Here's how the part is built. I have some questions about the finished solid (model axes, mm). A direction names the side the tool comes from. Round coordinates to 2 decimals unless told otherwise and drop trailing zeros. Order: outer loops, then holes, each group sorted by start corner. A loop starts at its lowest first (then second) coordinate and runs counter-clockwise, first axis right, second up.
Solid Edge part; units mm, degrees
sketch "Sketch1" plane through (0, 0, 0) normal (0, 0, 1) x (1, 0, 0)
  arc A0 (-0.5843, 4.4447) -> (0, 5.0777) centre (0.0507, 4.4447) cw
  arc A1 (0.5843, 4.4447) -> (0, 5.0777) centre (-0.0507, 4.4447) ccw
  line L0 (0.5843, 3.7649) -> (0.5843, 4.4447)
  arc A2 (2.249, 3.0754) -> (0.5843, 3.7649) centre (0, 0) ccw
  line L1 (2.249, 3.0754) -> (2.7297, 3.5561)
  arc A3 (2.7297, 3.5561) -> (3.5905, 3.5905) centre (3.1787, 3.1071) cw
  arc A4 (3.5561, 2.7297) -> (3.5905, 3.5905) centre (3.1071, 3.1787) ccw
  line L2 (3.0754, 2.249) -> (3.5561, 2.7297)
  arc A5 (3.7649, 0.5843) -> (3.0754, 2.249) centre (0, 0) ccw
  line L3 (3.7649, 0.5843) -> (4.4447, 0.5843)
  arc A6 (4.4447, 0.5843) -> (5.0777, 0) centre (4.4447, -0.0507) cw
  arc A7 (4.4447, -0.5843) -> (5.0777, 0) centre (4.4447, 0.0507) ccw
  line L4 (3.7689, -0.5843) -> (4.4447, -0.5843)
  line L5 (3.7625, -0.5998) -> (3.7689, -0.5843)
  arc A8 (3.7625, -0.5998) -> (3.0754, -2.249) centre (0, 0) cw
  line L6 (3.0754, -2.249) -> (3.5561, -2.7297)
  arc A9 (3.5561, -2.7297) -> (3.5905, -3.5905) centre (3.1071, -3.1787) cw
  arc A10 (2.7297, -3.5561) -> (3.5905, -3.5905) centre (3.1787, -3.1071) ccw
  line L7 (2.249, -3.0754) -> (2.7297, -3.5561)
  arc A11 (2.249, -3.0754) -> (0.5843, -3.7649) centre (0, 0) cw
  line L8 (0.5843, -3.7649) -> (0.5843, -4.4447)
  arc A12 (0.5843, -4.4447) -> (0, -5.0777) centre (-0.0507, -4.4447) cw
  arc A13 (-0.5843, -4.4447) -> (0, -5.0777) centre (0.0507, -4.4447) ccw
  line L9 (-0.5843, -3.7649) -> (-0.5843, -4.4447)
  arc A14 (-0.5843, -3.7649) -> (-2.249, -3.0754) centre (0, 0) cw
  line L10 (-2.249, -3.0754) -> (-2.7297, -3.5561)
  arc A15 (-2.7297, -3.5561) -> (-3.5905, -3.5905) centre (-3.1787, -3.1071) cw
  arc A16 (-3.5561, -2.7297) -> (-3.5905, -3.5905) centre (-3.1071, -3.1787) ccw
  line L11 (-3.0754, -2.249) -> (-3.5561, -2.7297)
  arc A17 (-3.0754, -2.249) -> (-3.7649, -0.5843) centre (0, 0) cw
  line L12 (-3.7649, -0.5843) -> (-4.4447, -0.5843)
  arc A18 (-4.4447, -0.5843) -> (-5.0777, 0) centre (-4.4447, 0.0507) cw
  arc A19 (-4.4447, 0.5843) -> (-5.0777, 0) centre (-4.4447, -0.0507) ccw
  line L13 (-3.7649, 0.5843) -> (-4.4447, 0.5843)
  arc A20 (-3.7649, 0.5843) -> (-3.0754, 2.249) centre (0, 0) cw
  line L14 (-3.0754, 2.249) -> (-3.5561, 2.7297)
  arc A21 (-3.5561, 2.7297) -> (-3.5905, 3.5905) centre (-3.1071, 3.1787) cw
  arc A22 (-2.7297, 3.5561) -> (-3.5905, 3.5905) centre (-3.1787, 3.1071) ccw
  line L15 (-2.249, 3.0754) -> (-2.7297, 3.5561)
  arc A23 (-2.249, 3.0754) -> (-0.5843, 3.7649) centre (0, 0) cw
  line L16 (-0.5843, 3.7649) -> (-0.5843, 4.4447)
extrude "Protrusion1" add sketch "Sketch1" along normal mid plane 6.35
sketch "Sketch2" plane through (0, 0, 0) normal (0, 0, 1) x (1, 0, 0)
  arc A0 (3.5561, 2.7297) -> (3.5905, 3.5905) centre (3.1071, 3.1787) ccw
  arc A1 (2.7297, 3.5561) -> (3.5905, 3.5905) centre (3.1787, 3.1071) cw
  arc A2 (3.5561, 2.7297) -> (2.7297, 3.5561) centre (3.1429, 3.1429) cw
  arc A3 (4.4447, 0.5843) -> (4.4447, -0.5843) centre (4.4447, 0) ccw
  arc A4 (4.4447, -0.5843) -> (5.0777, 0) centre (4.4447, 0.0507) ccw
  arc A5 (4.4447, 0.5843) -> (5.0777, 0) centre (4.4447, -0.0507) cw
  arc A6 (3.5561, -2.7297) -> (2.7297, -3.5561) centre (3.1429, -3.1429) ccw
  arc A7 (2.7297, -3.5561) -> (3.5905, -3.5905) centre (3.1787, -3.1071) ccw
  arc A8 (3.5561, -2.7297) -> (3.5905, -3.5905) centre (3.1071, -3.1787) cw
  arc A9 (0.5843, -4.4447) -> (0, -5.0777) centre (-0.0507, -4.4447) cw
  arc A10 (-0.5843, -4.4447) -> (0, -5.0777) centre (0.0507, -4.4447) ccw
  arc A11 (0.5843, -4.4447) -> (-0.5843, -4.4447) centre (0, -4.4447) ccw
  arc A12 (-2.7297, -3.5561) -> (-3.5561, -2.7297) centre (-3.1429, -3.1429) ccw
  arc A13 (-3.5561, -2.7297) -> (-3.5905, -3.5905) centre (-3.1071, -3.1787) ccw
  arc A14 (-2.7297, -3.5561) -> (-3.5905, -3.5905) centre (-3.1787, -3.1071) cw
  arc A15 (-4.4447, 0.5843) -> (-4.4447, -0.5843) centre (-4.4447, 0) cw
  arc A16 (-4.4447, -0.5843) -> (-5.0777, 0) centre (-4.4447, 0.0507) cw
  arc A17 (-4.4447, 0.5843) -> (-5.0777, 0) centre (-4.4447, -0.0507) ccw
  arc A18 (-2.7297, 3.5561) -> (-3.5905, 3.5905) centre (-3.1787, 3.1071) ccw
  arc A19 (-3.5561, 2.7297) -> (-3.5905, 3.5905) centre (-3.1071, 3.1787) cw
  arc A20 (-2.7297, 3.5561) -> (-3.5561, 2.7297) centre (-3.1429, 3.1429) cw
  arc A21 (0.5843, 4.4447) -> (-0.5843, 4.4447) centre (0, 4.4447) cw
  arc A22 (-0.5843, 4.4447) -> (0, 5.0777) centre (0.0507, 4.4447) cw
  arc A23 (0.5843, 4.4447) -> (0, 5.0777) centre (-0.0507, 4.4447) ccw
extrude "ExtrudedProtrusion_2" add sketch "Sketch2" against normal blind 4.445
sketch "Sketch3" plane through (0, 0, -3.175) normal (0, 0, -1) x (0, 1, 0)
  circle A0 centre (0, 0) radius 0.2794
extrude "Cutout1" cut sketch "Sketch3" against normal blind 26.4035
1. I'm going to push flat-ended pins straight in: P1, Ø1.5, axis at y = 4, z = -1.5, coming from the -X side; P2, Ø1.5, axis at x = 1, z = -0.5, coming from the -Y side; P3, Ø0.5, axis at y = -4.5, z = 0, coming from the +X side. Where does each tip first touch, or does it pass through?
Evaluation:
P1: stops at x = -3.74
P2: stops at y = -5
P3: stops at x = 0.58
2. If we section it at C-C, the plane y = -2: Write out the boundary of the cut face in (x, z) (3 decimals), and give its area (3 significant figures).
Evaluation:
outline: (-3.243, -3.175) - (3.243, -3.175) - (3.243, 3.175) - (-3.243, 3.175) - close
area: 41.2 mm2
3. If we section it at A-A, the plane y = 3.25: Write out the boundary of the cut face in (x, z) (3 decimals).
Evaluation:
outline: (-3.738, -4.445) - (-2.568, -4.445) - (-2.568, -3.175) - (-2.424, -3.175) - (-2.424, 3.175) - (-3.738, 3.175) - close; (-1.988, -3.175) - (1.988, -3.175) - (1.988, 3.175) - (-1.988, 3.175) - close; (2.424, -3.175) - (2.568, -3.175) - (2.568, -4.445) - (3.738, -4.445) - (3.738, 3.175) - (2.424, 3.175) - close
4. I need wall thicknesses on probe 1 along X at (y, z) = (0, -1.5); probe 2 along Z at (x, y) = (2.5, 2.5) (3 decimals); probe 3 along X at (y, z) = (4.5, -1.5). Which ranges of each line are inside material? Lowest first, please.
Evaluation:
probe 1: x = -5.08 to -0.28, 0.28 to 5.08
probe 2: z = -3.175 to 3.175
probe 3: x = -0.58 to 0.58
5. If we mould it in two halves opening along Y, with no side actions, what happens to faces 4 (the cylindrical face through (-3.74, 3.15, -0.69)), 5 (the cylindrical face through (3.86, 0.01, -3.8)), 6 (the flat face through (-3, -3, -4.445))? For each: released by +Y, released by -Y, zero draft, split by the parting line, or undercut.
Evaluation:
face 4: undercut
face 5: split by the parting line
face 6: zero draft
6. On a 3-axis mill with a long thin cutter (end or side, diameter ignored), from which of +Z, -Z, +X, -X, +Y, -Y can I reach the whole of each face in a straight line? I mean faces 1 (the cylindrical face through (-2.74, 2.72, -3.8)), 2 (the cylindrical face through (-1.47, 3.515, -0.044)), 3 (the cylindrical face through (-1.446, -3.525, -0.044)). Say none if no direction works.
Evaluation:
face 1: -Z
face 2: +Z, -Z, +Y
face 3: +Z, -Z, -Y
7. If we section it at B-B, the plane x = 4: Write out the boundary of the cut face in (y, z) (3 decimals), and give its area (3 significant figures).
Evaluation:
outline: (-0.584, -3.175) - (-0.379, -3.175) - (-0.379, -4.445) - (0.379, -4.445) - (0.379, -3.175) - (0.584, -3.175) - (0.584, 3.175) - (-0.584, 3.175) - close
area: 8.38 mm2
